Autodesk Inventor part; units mm, degrees
ref_plane "YZ Plane" through (0, 0, 0) normal (1, 0, 0) x (0, 1, 0)
ref_plane "XZ Plane" through (0, 0, 0) normal (0, 1, 0) x (-1, 0, 0)
ref_plane "XY Plane" through (0, 0, 0) normal (0, 0, 1) x (1, 0, 0)
sketch "Sketch1" plane through (0, 0, 0) normal (0, 0, 1) x (1, 0, 0)
  line L0 (-26.9235, 18.928) -> (13.0765, 18.928)
  line L1 (13.0765, 18.928) -> (13.0765, -11.072)
  line L2 (13.0765, -11.072) -> (-26.9235, -11.072)
  line L3 (-26.9235, -11.072) -> (-26.9235, 18.928)
  point P0 (0, 0)
  dimension "d1" = 30
  dimension "d47" = 40
extrude "Extrusion1" add sketch "Sketch1" along normal blind 10
sketch "Sketch2" plane through (13.0765, -11.072, 10) normal (1, 0, 0) x (0, 0, -1)
  line L0 (10, 30) -> (0, 30)
  line L1 (0, 0) -> (0, 30)
  line L2 (10, 0) -> (0, 0)
  circle A0 centre (-0.2, 15) radius 4.025
  line L3 (10, 30) -> (10, 0)
  dimension "d20" = 30
  dimension "d21" = 15
  dimension "d22" = 0.2
  dimension "d23" = 8.05
extrude "Extrusion3" cut sketch "Sketch2" against normal through all contours A0 L1 | L1 A0
sketch "Sketch3" plane through (0, 0, 10) normal (0, 0, 1) x (1, 0, 0)
  line L0 (13.0765, -0.092) -> (-26.9235, -0.092)
  line L1 (-26.9235, -0.092) -> (-26.9235, -11.072)
  line L2 (-26.9235, -11.072) -> (13.0765, -11.072)
  line L3 (13.0765, -11.072) -> (13.0765, -0.092)
  line L4 (-26.9235, 7.948) -> (13.0765, 7.948)
  line L5 (13.0765, 7.948) -> (13.0765, 18.928)
  line L6 (13.0765, 18.928) -> (-26.9235, 18.928)
  line L7 (-26.9235, 18.928) -> (-26.9235, 7.948)
  point P0 (0, 0)
  point P1 (8.5765, -5.582)
  point P2 (-22.4235, -5.582)
  point P3 (8.5765, 13.438)
  point P4 (-22.4235, 13.438)
  dimension "d26" = 4.5
  dimension "d27" = 10.98
  dimension "d28" = 5.49
  dimension "d29" = 5.49
  dimension "d30" = 4.5
hole "Hole2" at (8.5765, -5.582, 10) at (-22.4235, -5.582, 10) at (8.5765, 13.438, 10) at (-22.4235, 13.438, 10) direction (0, 0, -1) diameter 3 depth 20 tip angle 118
fillet "Fillet2" radius 0.5 4 edges at (13.0765, 18.928, 5) (-26.9235, 18.928, 5) (13.0765, -11.072, 5) (-26.9235, -11.072, 5)
sketch "Sketch5" plane through (0, 0, 0) normal (0, 0, -1) x (-1, 0, 0)
  arc A0 (26.4235, -11.072) -> (26.9235, -10.572) centre (26.4235, -10.572) ccw
  line L0 (26.9235, -10.572) -> (26.9235, 18.428)
  arc A1 (26.9235, 18.428) -> (26.4235, 18.928) centre (26.4235, 18.428) ccw
  line L1 (26.4235, 18.928) -> (-12.5765, 18.928)
  arc A2 (-12.5765, 18.928) -> (-13.0765, 18.428) centre (-12.5765, 18.428) ccw
  line L2 (-13.0765, 18.428) -> (-13.0765, -10.572)
  arc A3 (-13.0765, -10.572) -> (-12.5765, -11.072) centre (-12.5765, -10.572) ccw
  line L3 (-12.5765, -11.072) -> (26.4235, -11.072)
  circle A4 centre (-8.5765, 13.438) radius 1.5
  circle A5 centre (-8.5765, -5.582) radius 1.5
  circle A6 centre (22.4235, -5.582) radius 1.5
  circle A7 centre (22.4235, 13.438) radius 1.5
  point P0 (0, 0)
  point P1 (10.9235, -6.822)
  point P2 (10.9235, 14.678)
  dimension "d48" = 4.25
  dimension "d49" = 4.25
  dimension "d50" = 16
hole "Hole4" at (-10.9235, -6.822, 0) at (-10.9235, 14.678, 0) direction (0, 0, 1) diameter 2.5 depth 8 tip angle 118
properties part number "3DP_PLA_Y_axis_linear_shaft_mount_clamp_with_endstop" material "ABS Plastic"
Work out the finished part from the listing and answer in its coordinate system (mm). A direction names the side the tool comes from. Coordinates: 2 decimals unless noted, no trailing zeros. Loops run counter-clockwise (first coordinate to the right, second up) from the corner with the lowest first, then second, coordinate; pieces in that order, holes last. Notation, with made-up numbers: M 82.5,-34 L 121.5,-34 A19 ccw 121.5,-5 Z; hole C -19.5,85.25 d2. An arc over 180 degrees is marked long. Use CSV: the item, a comma, the result in double quotes. Start each with the question number.
(1) For faces 4 (the face through (-11.978, 15.35, 4.056)), 5 (the face through (9.91, 12.75, 4.93)), determine the directions among +Z, -Z, +X, -X, +Y, -Y from which every point of the face is accessible in a straight line to the end or side of a thin tool.
(2) Given pin 1 Ø5 at (x, y) = (-22.42, 13.44) entering from +Z; pin 2 Ø2 at (x, y) = (-10.92, 14.68) entering from -Z, each flat-ended and moving along its own axis, determine where each tip first touches the part or whether it passes through.
(3) Consider line 1 (X direction, y = -5.5, z = 9); line 2 (X direction, y = 13, z = 7.5); line 3 (X direction, y = 14.75, z = 6.25). Determine where each line is inside the solid, lowest interval first.
(4) Find section A-A, the plane z = 9.25. Give the vertices of the cut face in (x, y).
(5) Find section D-D, the plane z = 4.75. Give the vertices of the cut face in (x, y), then the cut area to 3 significant figures.
(6) For a pull along Y with two mould halves and no side action, classify faces 1 (the face through (-6.643, 3.842, 6.176)), 2 (the face through (-7, 18.928, 5)), 3 (the face through (-7, 14, 10)) as +Y half, -Y half, draft (parallel to the pull), parting line (faces both ways), or undercut.
(7) Find section B-B, the plane z = 6.75. Give the vertices of the cut face in (x, y).
(8) Find section C-C, the plane y = 12.75. Give the vertices of the cut face in (x, z).
Recorded:
1,face 4,"-Z"
1,face 5,"+Z, -Z"
2,pin 1,"stops at z = 10"
2,pin 2,"stops at z = 8.15"
3,line 1,"x = -26.92 to -23.92, -20.93 to 7.08, 10.07 to 13.08"
3,line 2,"x = -26.92 to -23.86, -20.99 to 7.14, 10.01 to 13.08"
3,line 3,"x = -26.92 to -23.15, -21.7 to -12.17, -9.68 to 7.85, 9.3 to 13.08"
4,outline,"M -26.92,-10.57 A0.5 ccw -26.42,-11.07 L 12.58,-11.07 A0.5 ccw 13.08,-10.57 L 13.08,0.02 L -26.92,0.02 Z; M -26.92,7.84 L 13.08,7.84 L 13.08,18.43 A0.5 ccw 12.58,18.93 L -26.42,18.93 A0.5 ccw -26.92,18.43 Z; hole C -22.42,-5.58 d3; hole C -22.42,13.44 d3; hole C 8.58,-5.58 d3; hole C 8.58,13.44 d3"
5,outline,"M -26.92,-10.57 A0.5 ccw -26.42,-11.07 L 12.58,-11.07 A0.5 ccw 13.08,-10.57 L 13.08,18.43 A0.5 ccw 12.58,18.93 L -26.42,18.93 A0.5 ccw -26.92,18.43 Z; hole C -22.42,-5.58 d3; hole C -22.42,13.44 d3; hole C -10.92,-6.82 d2.5; hole C -10.92,14.68 d2.5; hole C 8.58,-5.58 d3; hole C 8.58,13.44 d3"
5,area,"1,160 mm^2"
6,face 1,"undercut"
6,face 2,"+Y half"
6,face 3,"draft"
7,outline,"M -26.92,-10.57 A0.5 ccw -26.42,-11.07 L 12.58,-11.07 A0.5 ccw 13.08,-10.57 L 13.08,1.85 L -26.92,1.85 Z; M -26.92,6 L 13.08,6 L 13.08,18.43 A0.5 ccw 12.58,18.93 L -26.42,18.93 A0.5 ccw -26.92,18.43 Z; hole C -22.42,-5.58 d3; hole C -22.42,13.44 d3; hole C -10.92,-6.82 d2.5; hole C -10.92,14.68 d2.5; hole C 8.58,-5.58 d3; hole C 8.58,13.44 d3"
8,outline,"M -26.92,0 L -23.76,0 L -23.76,10 L -26.92,10 Z; M -21.09,0 L 7.24,0 L 7.24,10 L -21.09,10 Z; M 9.91,0 L 13.08,0 L 13.08,10 L 9.91,10 Z"
